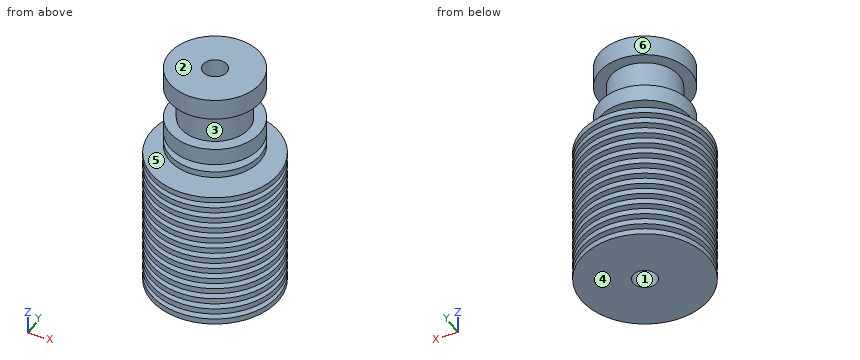
```python
from build123d import *

# Parameters (mm, degrees)
F3_D = 4.2


with BuildPart() as f1:
    # F0 (on Front) → F1 (revolve)
    with BuildSketch(Plane.XZ):
        Polygon((8, 0), (0, 0), (0, -41.7), (11.2, -41.7), (11.2, -16.7), (4.193673376, -16.7), (4.193673376, -15.2441602767), (8, -15.2441602767), (8, -14.1522795528), (4.193673376, -14.1522795528), (4.193673376, -12.7), (8, -12.7), (8, -9.7), (6, -9.7), (6, -3.7), (8, -3.7), align=None)
    revolve(axis=Axis((0, 0, -23.3692955226), (0, 0, -1)))

    # F3 (through all)
    with Locations(Plane(origin=(0, 0, -41.7), x_dir=(1, 0, 0), z_dir=(0, 0, -1))):
        with Locations((0, 0)):
            Hole(F3_D / 2)

    # F4 (on Front) → F5 (revolve, cut)
    with BuildSketch(Plane.XZ):
        Polygon((11.2, -18.7), (11.2, -17.7), (3.5, -17.7), (3.6304347826, -18.7), align=None)
        Polygon((11.2, -39.7), (6.3695652174, -39.7), (6.5, -40.7), (11.2, -40.7), align=None)
        Polygon((11.2, -37.7), (6.1086956522, -37.7), (6.2391304348, -38.7), (11.2, -38.7), align=None)
        Polygon((11.2, -35.7), (5.847826087, -35.7), (5.9782608696, -36.7), (11.2, -36.7), align=None)
        Polygon((11.2, -33.7), (5.5869565217, -33.7), (5.7173913043, -34.7), (11.2, -34.7), align=None)
        Polygon((11.2, -31.7), (5.3260869565, -31.7), (5.4565217391, -32.7), (11.2, -32.7), align=None)
        Polygon((11.2, -29.7), (5.0652173913, -29.7), (5.1956521739, -30.7), (11.2, -30.7), align=None)
        Polygon((11.2, -27.7), (4.8043478261, -27.7), (4.9347826087, -28.7), (11.2, -28.7), align=None)
        Polygon((11.2, -25.7), (4.5434782609, -25.7), (4.6739130435, -26.7), (11.2, -26.7), align=None)
        Polygon((11.2, -23.7), (4.2826086957, -23.7), (4.4130434783, -24.7), (11.2, -24.7), align=None)
        Polygon((11.2, -21.7), (4.0217391304, -21.7), (4.152173913, -22.7), (11.2, -22.7), align=None)
        Polygon((11.2, -19.7), (3.7608695652, -19.7), (3.8913043478, -20.7), (11.2, -20.7), align=None)
    revolve(axis=Axis((0, 0, -17.9993046731), (0, 0, -1)), mode=Mode.SUBTRACT)


solid = f1.part
```
Can you work these out from the model? Positions are in its coordinate system, mm. Face numbers are marked on the shaded views. A direction names the side the tool comes from. Round coordinates to 2 decimals unless told otherwise and drop trailing zeros. Loops run counter-clockwise (first coordinate to the right, second up) from the corner with the lowest first, then second, coordinate; pieces in that order, holes last. Notation, with made-up numbers: (-40, 28) -> (-2, 28) arc R19 ccw to (-2, 37) -> close; hole circle Ø4 at (65, 71.25). An arc over 180 degrees is marked (long way). One line per item, written item: value. Start each with the question number.
1. If I drill on probe 1 along Y at (x, z) = (0, -29); probe 2 along Y at (x, z) = (1.25, -12); probe 3 along X at (y, z) = (-0.25, -9.5), over which ranges is the centre line in solid material (lowest first)?
2. For the marked faces 4, 5 and 6, which set-ups out of +Z, -Z, +X, -X, +Y, -Y let a thin tool reach every point of the face, with its end or its side?
3. If we section it at A-A, the plane z = -6.5: Write out the boundary of the cut face in (x, y).
4. If we section it at B-B, the plane x = 7: Give the number of separate pieces and of enclosed holes in the cut face, then the cut area to 3 significant figures.
5. For pin 1 (6 mm diameter, centred on y = -6, z = -5, fed in from -X); pin 2 (5 mm diameter, centred on x = -6, z = -9, fed in from +Y); pin 3 (1 mm diameter, centred on y = 2.5, z = -21, fed in from +X), each with a flat end and sliding along its axis, tell me the tip position at first contact or that it passes through.
6. If we mould it in two halves opening along X, with no side actions, what happens to the marked faces 1, 2 and 3? For each: pulls with the +X half, pulls with the -X half, needs draft (parallel to the pull), parting line crosses it, or undercut.
Calculated:
1. probe 1: y = -11.2 to -2.1, 2.1 to 11.2
1. probe 2: y = -7.9 to -1.69, 1.69 to 7.9
1. probe 3: x = -5.99 to -2.09, 2.09 to 5.99
2. face 4: -Z, +X, -X, +Y, -Y
2. face 5: none
2. face 6: +Z
3. outline: circle Ø12 at (0, 0); hole circle Ø4.2 at (0, 0)
4. separate pieces: 16
4. enclosed holes: 0
4. area: 288 mm²
5. pin 1: stops at x = -7.29
5. pin 2: stops at y = 7.14
5. pin 3: stops at x = 11.02
6. face 1: undercut
6. face 2: needs draft
6. face 3: parting line crosses it
